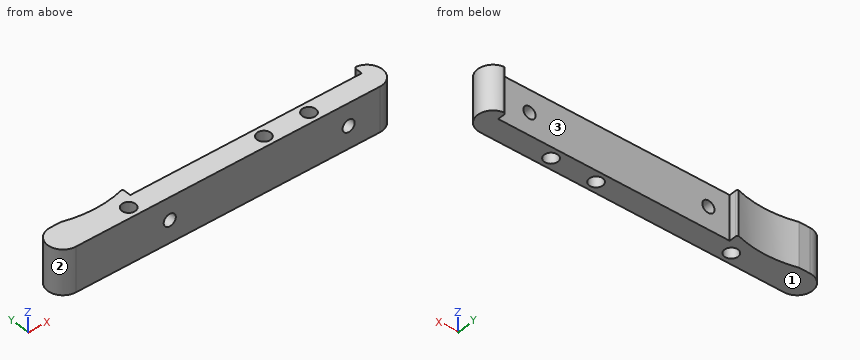
from build123d import *

# Parameters (mm, degrees)
SKETCH1_R           = 2.413
BOSS_EXTRUDE1_DEPTH = 15.8242
SKETCH3_R           = 2.159
CUT_EXTRUDE1_DEPTH  = 7.62
CUT_EXTRUDE2_DEPTH  = 15.8242
FILLET1_R           = 0.762


with BuildPart() as part:
    # Sketch1 → Boss-Extrude1 (new body)
    with BuildSketch(Plane.XY):
        with BuildLine():
            Line((0, 0), (107.95, 0))
            ThreePointArc((107.95, 0), (113.3602, 5.4102), (107.95, 10.8204))
            Line((107.95, 10.8204), (107.95, 7.62))
            Line((107.95, 7.62), (25.781, 7.62))
            Line((25.781, 7.62), (25.781, 10.8204))
            Line((25.781, 10.8204), (0, 10.8204))
            ThreePointArc((0, 10.8204), (-5.4102, 5.4102), (0, 0))
        make_face()
        with Locations((21.971, 3.81)):
            Circle(SKETCH1_R, mode=Mode.SUBTRACT)
        with Locations((69.977, 3.81)):
            Circle(SKETCH1_R, mode=Mode.SUBTRACT)
        with Locations((85.979, 3.81)):
            Circle(SKETCH1_R, mode=Mode.SUBTRACT)
    extrude(amount=BOSS_EXTRUDE1_DEPTH)

    # Sketch3 → Cut-Extrude1 (cut)
    with BuildSketch(Plane(origin=(0, 7.62, 0), x_dir=(1, 0, 0), z_dir=(0, 1, 0))):
        with Locations(Location((96.8375, -7.9121, 0), (0, 0, 270))):
            Circle(SKETCH3_R)
        with Locations(Location((33.3375, -7.9121, 0), (0, 0, 270))):
            Circle(SKETCH3_R)
    extrude(amount=-CUT_EXTRUDE1_DEPTH, mode=Mode.SUBTRACT)

    # Sketch4 → Cut-Extrude2 (cut)
    with BuildSketch(Plane(origin=(0, 0, 0), x_dir=(-1, 0, 0), z_dir=(0, 0, -1))):
        with BuildLine():
            Line((-3.81, 10.8204), (-25.4, 10.8204))
            ThreePointArc((-25.4, 10.8204), (-14.605, 9.241326758), (-3.81, 10.8204))
        make_face()
    extrude(amount=-CUT_EXTRUDE2_DEPTH, mode=Mode.SUBTRACT)

    # Fillet1
    # the kernel refuses this fillet: 0.762 mm, written as the material it takes off along each edge
    with BuildSketch(Plane(origin=(107.95, 10.8204, -2.224832658), x_dir=(0.9966120705297453, -0.08224585627503565, 0), z_dir=(0, 0, 1))) as fillet1_piece_1:
        with BuildLine():
            CenterArc((0.827261721, -0.759418398), FILLET1_R, 85.282330638, 99.435338723)
            Line((0.067843323, -0.82208974), (0.052654955, -0.823343167))
            Line((0.052654955, -0.823343167), (-0.015188368, -0.001253427))
            Line((-0.015188368, -0.001253427), (-0.001253427, 0.015188368))
            ThreePointArc((-0.001253427, 0.015188368), (0.444966532, 0.033569376), (0.89118649, 0.015188368))
            Line((0.89118649, 0.015188368), (0.889933063, 0))
        make_face()
    extrude(amount=20.273865316, mode=Mode.SUBTRACT)
    with BuildSketch(Plane(origin=(25.781, 10.8204, -1.649778394), x_dir=(-1, 0, 0), z_dir=(0, 0, 1))) as fillet1_piece_2:
        with BuildLine():
            CenterArc((0.762, 0.659911358), FILLET1_R, 180, 60)
            Line((0, 0.659911358), (-0.01524, 0.659911358))
            Line((-0.01524, 0.659911358), (-0.01524, 0))
            Line((-0.01524, 0), (0, -0.01524))
            ThreePointArc((0, -0.01524), (0.1905, -0.01524), (0.37338, -0.013198227))
            Line((0.37338, -0.013198227), (0.381, 0))
        make_face()
    extrude(amount=19.123756788, mode=Mode.SUBTRACT)


solid = part.part
CAD build for the part. Positions are in the model's coordinates, mm. Face numbers are marked on the shaded views. Round coordinates to 2 decimals unless told otherwise and drop trailing zeros. Write each loop counter-clockwise with the first axis right and the second up, starting at its lowest first coordinate (ties: lowest second). Pieces come first, ordered by that corner, then holes.
(1) Slice it at A-A, the plane z = 9. Write the cut outline in (x, y) (3 decimals), and give its area (3 significant figures).
(2) Slice it at D-D, the plane x = 42.5. Write the cut outline in (y, z), and give its area (3 significant figures).
(3) Slice it at B-B, the plane y = 3.81. Write the cut outline in (x, z).
(4) Slice it at C-C, the plane z = 4.75. Write the cut outline in (x, y) (3 decimals), and give its area (3 significant figures).
(5) Mould opens along X. For the marked faces 1, 2 and 3 say: pulls with the +X half, pulls with the -X half, needs draft (parallel to the pull), parting line crosses it, or undercut.
(6) Drop flat-ended pins along their axis: P1, Ø5, axis at y = 2, z = 12, coming from the -X side; P2, Ø0.7, axis at y = 9, z = 6, coming from the -X side; P3, Ø1.3, axis at y = 9, z = 11.5, coming from the +X side. Give the stop position or say it passes through.
(7) Probe line 1 along X through (y, z) = (7.5, 8.75); line 2 along X through (y, z) = (6.75, 9); line 3 along X through (y, z) = (5, 2). List the from-to ranges inside material, lowest first.
From the geometry:
1. outline: (0, 0) - (31.473, 0) - (31.473, 7.62) - (25.781, 7.62) - (25.781, 10.16) arc R0.762 ccw to (25.4, 10.82) arc R37.688 cw to (3.81, 10.82) - (0, 10.82) arc R5.41 ccw to start; (35.202, 0) - (94.973, 0) - (94.973, 7.62) - (35.202, 7.62) - close; (98.702, 0) - (107.95, 0) arc R5.41 ccw to (108.837, 10.747) arc R0.762 ccw to (107.95, 9.996) - (107.95, 7.62) - (98.702, 7.62) - close; hole circle Ø4.826 at (21.971, 3.81); hole circle Ø4.826 at (69.977, 3.81); hole circle Ø4.826 at (85.979, 3.81)
1. area: 862 mm2
2. outline: (0, 0) - (7.62, 0) - (7.62, 15.82) - (0, 15.82) - close
2. area: 121 mm2
3. outline: (-5.17, 0) - (19.56, 0) - (19.56, 15.82) - (-5.17, 15.82) - close; (24.38, 0) - (67.56, 0) - (67.56, 15.82) - (24.38, 15.82) - close; (72.39, 0) - (83.57, 0) - (83.57, 15.82) - (72.39, 15.82) - close; (88.39, 0) - (113.12, 0) - (113.12, 15.82) - (88.39, 15.82) - close; hole circle Ø4.32 at (33.34, 7.91); hole circle Ø4.32 at (96.84, 7.91)
4. outline: (0, 0) - (107.95, 0) arc R5.41 ccw to (108.837, 10.747) arc R0.762 ccw to (107.95, 9.996) - (107.95, 7.62) - (25.781, 7.62) - (25.781, 10.16) arc R0.762 ccw to (25.4, 10.82) arc R37.688 cw to (3.81, 10.82) - (0, 10.82) arc R5.41 ccw to start; hole circle Ø4.826 at (21.971, 3.81); hole circle Ø4.826 at (69.977, 3.81); hole circle Ø4.826 at (85.979, 3.81)
4. area: 919 mm2
5. face 1: needs draft
5. face 2: pulls with the -X half
5. face 3: undercut
6. P1: stops at x = -5.33
6. P2: stops at x = -4.33
6. P3: stops at x = 112.49
7. line 1: x = -4.99 to 31.35, 35.33 to 94.85, 98.83 to 112.94
7. line 2: x = -5.24 to 31.47, 35.2 to 94.97, 98.7 to 113.19
7. line 3: x = -5.39 to 19.87, 24.07 to 67.88, 72.08 to 83.88, 88.08 to 113.34
